Source: CAD feature listing. Evaluate the final solid. Frame: model axes, mm. A direction names the side the tool comes from. Give positions to 0.01 mm unless a question says otherwise; leave off trailing zeros. Loops run counter-clockwise (first coordinate to the right, second up) from the corner with the lowest first, then second, coordinate; pieces in that order, holes last. Notation, with made-up numbers: (-12, -34) -> (16, -34) arc R15 cw to (16, -29) -> close; hole circle Ø8 at (-32.5, 44). An arc over 180 degrees is marked (long way). Return JSON: item names as keys, results as strings. Group by question number.
```python
from build123d import *

# Parameters (mm, degrees)
EXTRUDE_1_DEPTH     = 25
SKETCH_2_R          = 1.5
SKETCH_2_R_2        = 4
CUT_EXTRUDE_1_DEPTH = 25
SKETCH_3_R          = 1.5
SKETCH_3_R_2        = 4
CUT_EXTRUDE_2_DEPTH = 25
FILLET_1_R          = 2


with BuildPart() as part:
    # 草图1 → 凸台-拉伸1 (new body)
    with BuildSketch(Plane(origin=(0, 0, 0), x_dir=(1, 0, 0), z_dir=(0, 1, 0))):
        Polygon((0, 0), (27.5, 0), (27.5, 64.5), (25.5, 64.5), (25.5, 2), (0, 2), align=None)
    extrude_1 = extrude(amount=EXTRUDE_1_DEPTH)

    # 草图2 → 切除-拉伸1 (cut)
    with BuildSketch(Plane(origin=(27.5, 0, 0), x_dir=(0, 0, -1), z_dir=(1, 0, 0))):
        with Locations((16.53, 12.5)):
            Circle(SKETCH_2_R)
        with Locations((45, 12.5)):
            Circle(SKETCH_2_R)
        with Locations((52, 12.5)):
            Circle(SKETCH_2_R_2)
        with Locations((52, 19.5)):
            Circle(SKETCH_2_R)
        with Locations((59, 12.5)):
            Circle(SKETCH_2_R)
        with Locations((52, 5.5)):
            Circle(SKETCH_2_R)
        with BuildLine():
            Line((64.5, 25), (52, 25))
            ThreePointArc((52, 25), (60.838834765, 21.338834765), (64.5, 12.5))
            Line((64.5, 12.5), (64.5, 25))
        make_face()
        with BuildLine():
            Line((64.5, 0), (64.5, 12.5))
            ThreePointArc((64.5, 12.5), (60.838834765, 3.661165235), (52, 0))
            Line((52, 0), (64.5, 0))
        make_face()
        with Locations((33.4, 12.5)):
            Circle(SKETCH_2_R)
    cut_extrude_1 = extrude(amount=-CUT_EXTRUDE_1_DEPTH, mode=Mode.SUBTRACT)

    # 镜向1: 凸台-拉伸1, 切除-拉伸1 across plane
    add(extrude_1.mirror(Plane(origin=(0, 25, -2), x_dir=(0, 0, 1), z_dir=(1, 0, 0))))
    add(cut_extrude_1.mirror(Plane(origin=(0, 25, -2), x_dir=(0, 0, 1), z_dir=(1, 0, 0))), mode=Mode.SUBTRACT)

    # 草图3 → 切除-拉伸2 (cut)
    with BuildSketch(Plane.XY):
        with Locations((7, 12.5)):
            Circle(SKETCH_3_R)
        with Locations((0, 19.5)):
            Circle(SKETCH_3_R)
        with Locations((-7, 12.5)):
            Circle(SKETCH_3_R)
        with Locations((0, 5.5)):
            Circle(SKETCH_3_R)
        with Locations((18.6, 12.5)):
            Circle(SKETCH_3_R)
        with Locations((-18.6, 12.5)):
            Circle(SKETCH_3_R)
        with Locations((0, 12.5)):
            Circle(SKETCH_3_R_2)
    extrude(amount=-CUT_EXTRUDE_2_DEPTH, mode=Mode.SUBTRACT)

    # 圆角1
    fillet_1_edges = [part.edges().sort_by_distance(p)[0] for p in [
        (25.5, 12.5, -2),
        (27.5, 12.5, 0),
        (-25.5, 12.5, -2),
        (-27.5, 12.5, 0),
    ]]
    fillet(fillet_1_edges, radius=FILLET_1_R)


solid = part.part
```
1) Contact query for flat-ended pins moving along their axis: P1, Ø7.5, axis at x = -7.5, y = 14.5, coming from the -Z side; P2, Ø2.5, axis at y = 19.5, z = -52, coming from the +X side. Output: stop coordinate, or through.
2) Cut plane A-A on x = 0. Return loops of the section in (y, z).
3) Cut plane D-D on x = 7. Return loops of the section in (y, z), then the cut area to 3 significant figures.
4) Material intervals for line 1 (Y direction, x = 0, z = -1); line 2 (X direction, y = 14.75, z = -38); line 3 (Z direction, x = -8, y = 15), sorted ascending.
5) Mould query, pull axis Y, two halves, no side actions, for faces 3 (the face through (26.514, 13.701, -55.815)), 4 (the face through (0, 0, -1)), 5 (the face through (24.93, 12.68, -2.6)). Classes: released by +Y, released by -Y, zero draft, split by the parting line, or undercut.
6) Cut plane B-B on z = -33.4. Return loops of the section in (x, y), then the cut area to 3 significant figures.
7) Reachability of faces 1 (the face through (-24.9, 12.68, -2.57)), 2 (the face through (26.9, 12.68, -0.57)) from +Z, -Z, +X, -X, +Y, -Y: full face, straight path, thin tool, end or side. Return the list, or none.
8) Cut plane C-C on z = -6.5. Return loops of the section in (x, y), then the cut area to 3 significant figures.
Calculated:
{
 "1": {"P1": "z = -2", "P2": "through"},
 "2": {"outline": "(0, -2) -> (4, -2) -> (4, 0) -> (0, 0) -> close; (7, -2) -> (8.5, -2) -> (8.5, 0) -> (7, 0) -> close; (16.5, -2) -> (18, -2) -> (18, 0) -> (16.5, 0) -> close; (21, -2) -> (25, -2) -> (25, 0) -> (21, 0) -> close"},
 "3": {"outline": "(0, -2) -> (11, -2) -> (11, 0) -> (0, 0) -> close; (14, -2) -> (25, -2) -> (25, 0) -> (14, 0) -> close", "area": "44.0 mm2"},
 "4": {"line 1": "0 to 4, 7 to 8.5, 16.5 to 18, 21 to 25", "line 2": "-27.5 to -25.5, 25.5 to 27.5", "line 3": "-2 to 0"},
 "5": {"face 3": "undercut", "face 4": "released by -Y", "face 5": "zero draft"},
 "6": {"outline": "(-27.5, 0) -> (-25.5, 0) -> (-25.5, 11) -> (-27.5, 11) -> close; (-27.5, 14) -> (-25.5, 14) -> (-25.5, 25) -> (-27.5, 25) -> close; (25.5, 0) -> (27.5, 0) -> (27.5, 11) -> (25.5, 11) -> close; (25.5, 14) -> (27.5, 14) -> (27.5, 25) -> (25.5, 25) -> close", "area": "88.0 mm2"},
 "7": {"face 1": "-Z, +Y, -Y", "face 2": "+Z, +X, +Y, -Y"},
 "8": {"outline": "(-27.5, 0) -> (-25.5, 0) -> (-25.5, 25) -> (-27.5, 25) -> close; (25.5, 0) -> (27.5, 0) -> (27.5, 25) -> (25.5, 25) -> close", "area": "100 mm2"}
}
